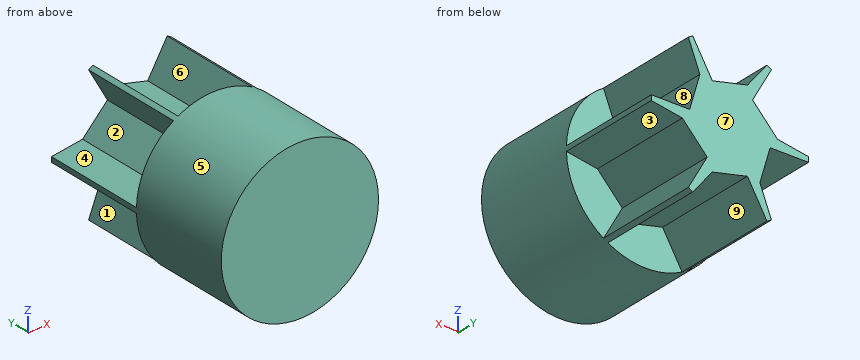
Autodesk Inventor part; units mm, degrees
ref_plane "YZ Plane" through (0, 0, 0) normal (1, 0, 0) x (0, 1, 0)
ref_plane "XZ Plane" through (0, 0, 0) normal (0, 1, 0) x (-1, 0, 0)
ref_plane "XY Plane" through (0, 0, 0) normal (0, 0, 1) x (1, 0, 0)
sketch "Sketch1" plane through (0, 0, 0) normal (0, 1, 0) x (-1, 0, 0)
  circle A0 centre (0, 0) radius 9.525
  dimension "d0" = 19.05
extrude "Extrusion1" add sketch "Sketch1" along normal blind 25.4
sketch "Sketch2" plane through (0, 25.4, 0) normal (0, 1, 0) x (1, 0, 0)
  arc A0 (4.4938, 8.3983) -> (-4.4938, 8.3983) centre (0, 0) ccw
  line L0 (-4.4938, 8.3983) -> (-2.1272, 4.4011)
  line L1 (-2.1272, 4.4011) -> (2.1272, 5.428)
  line L2 (2.1272, 5.428) -> (4.4938, 8.3983)
extrude "Extrusion2" cut sketch "Sketch2" against normal blind 12.7
pattern_circular "Circular Pattern1" count 6 over 360 about axis through (0, -10, 0) along (0, 1, 0) of "Extrusion2"
properties part number "test"
CAD build for the part. Positions are in the model's coordinates, mm. Face numbers are marked on the shaded views. A direction names the side the tool comes from. Give positions to 0.01 mm unless a question says otherwise; leave off trailing zeros. Write each loop counter-clockwise with the first axis right and the second up, starting at its lowest first coordinate (ties: lowest second). Pieces come first, ordered by that corner, then holes. Notation, with made-up numbers: (46, 42) -> (93, 42) arc R20 ccw to (93, 50) -> close; hole circle Ø10 at (8, 64.25). An arc over 180 degrees is marked (long way). Return JSON: item names as keys, results as strings.
Item 1: Drill centre lines: probe 1 along Y at (x, z) = (5, 2.5); probe 2 along X at (y, z) = (6, 4.5); probe 3 along X at (y, z) = (16.5, 2.5). Where is each one in solid material? Low to high.
Answer below:
{"probe 1": "y = 0 to 12.7", "probe 2": "x = -8.39 to 8.39", "probe 3": "x = -4.22 to 4.24"}
Item 2: Drop flat-ended pins along their axis: pin 1 (1.5 mm diameter, centred on x = 6, z = 2, fed in from +Y); pin 2 (1 mm diameter, centred on y = 22, z = 5.5, fed in from -X); pin 3 (1 mm diameter, centred on x = 6, y = 4, fed in from -Z). Give the stop position or say it passes through.
Answer below:
{"pin 1": "stops at y = 12.7", "pin 2": "stops at x = -3.85", "pin 3": "stops at z = -7.78"}
Item 3: Two-plate mould, pull along Z, no slides. Class the marked faces 1, 2, 3 and 4: +Z half, -Z half, draft (parallel to the pull), parting line (faces both ways), or undercut.
Answer below:
{"face 1": "undercut", "face 2": "undercut", "face 3": "-Z half", "face 4": "+Z half"}
Item 4: Band-saw the part on D-D (x = -7.25). List the corners of the cut face in (y, z).
Answer below:
{"outline": "(0, -6.18) -> (12.7, -6.18) -> (12.7, -0.33) -> (25.4, -0.33) -> (25.4, 0.65) -> (12.7, 0.65) -> (12.7, 6.18) -> (0, 6.18) -> close"}
Item 5: Tool access for the marked faces 5, 6, 7, 8 and 9: list every direction of +Z, -Z, +X, -X, +Y, -Y with a clear straight run to the whole face (end or side of a thin tool).
Answer below:
{"face 5": "+Y, -Y", "face 6": "+Z, +Y", "face 7": "+Z, -Z, +X, -X, +Y", "face 8": "+X, +Y", "face 9": "-Z, +Y"}
Item 6: Band-saw the part on A-A (y = 17). List the corners of the cut face in (x, z) (3 decimals).
Answer below:
{"outline": "(-9.52, -0.307) -> (-4.875, -0.358) -> (-3.637, -4.556) -> (-5.026, -8.091) arc R9.525 ccw to (-4.494, -8.398) -> (-2.127, -4.401) -> (2.127, -5.428) -> (4.494, -8.398) arc R9.525 ccw to (5.026, -8.091) -> (2.748, -4.043) -> (5.764, -0.872) -> (9.52, -0.307) arc R9.525 ccw to (9.52, 0.307) -> (4.875, 0.358) -> (3.637, 4.556) -> (5.026, 8.091) arc R9.525 ccw to (4.494, 8.398) -> (2.127, 4.401) -> (-2.127, 5.428) -> (-4.494, 8.398) arc R9.525 ccw to (-5.026, 8.091) -> (-2.748, 4.043) -> (-5.764, 0.872) -> (-9.52, 0.307) arc R9.525 ccw to start"}
Item 7: Band-saw the part on B-B (x = 0). List the corners of the cut face in (y, z) (3 decimals).
Answer below:
{"outline": "(0, -9.525) -> (12.7, -9.525) -> (12.7, -4.915) -> (25.4, -4.915) -> (25.4, 4.915) -> (12.7, 4.915) -> (12.7, 9.525) -> (0, 9.525) -> close"}
Item 8: Band-saw the part on C-C (z = 7). List the corners of the cut face in (x, y), then the cut area to 3 significant figures.
Answer below:
{"outline": "(-6.46, 0) -> (6.46, 0) -> (6.46, 12.7) -> (4.6, 12.7) -> (4.6, 25.4) -> (3.67, 25.4) -> (3.67, 12.7) -> (-3.38, 12.7) -> (-3.38, 25.4) -> (-4.41, 25.4) -> (-4.41, 12.7) -> (-6.46, 12.7) -> close", "area": "189 mm2"}
